Geometry check sheet. Reference: the model listing, model coordinates, mm. Face numbers are marked on the shaded views. A direction names the side the tool comes from. Coordinates: 2 decimals unless noted, no trailing zeros. Loops run counter-clockwise (first coordinate to the right, second up) from the corner with the lowest first, then second, coordinate; pieces in that order, holes last. Notation, with made-up numbers: M 63,13.25 L 119,13.25 A27 ccw 119,37.25 Z; hole C 53,-19.5 d11. An arc over 180 degrees is marked long. One line per question, with ' | ' between items. Start each with the question number.
from build123d import *

# Parameters (mm, degrees)
ESQUISSE1_R                  = 5
BOSS_EXTRU_1_DEPTH           = 10
ENL_V_MAT_EXTRU_1_DEPTH      = 3
ESQUISSE3_R                  = 2.65
ENL_V_MAT_EXTRU_2_DEPTH      = 6
ENL_V_MAT_EXTRU_3_DEPTH      = 13.247448714
ENL_V_MAT_EXTRU_3_DEPTH_BACK = 13.247448714
ESQUISSE4_R                  = 1.5
ESQUISSE5_R                  = 2.65
ENL_V_MAT_EXTRU_4_DEPTH      = 10.273618668


with BuildPart() as part:
    # Esquisse1 → Boss.-Extru.1 (new body)
    with BuildSketch(Plane.XY):
        Circle(ESQUISSE1_R)
    extrude(amount=BOSS_EXTRU_1_DEPTH)

    # Esquisse2 → Enlèv. mat.-Extru.1 (cut)
    with BuildSketch(Plane.XY.offset(10)):
        Polygon((3.7, -2.136195996), (3.7, 2.136195996), (0, 4.272391992), (-3.7, 2.136195996), (-3.7, -2.136195996), (0, -4.272391992), align=None)
    extrude(amount=-ENL_V_MAT_EXTRU_1_DEPTH, mode=Mode.SUBTRACT)

    # Esquisse3 → Enlèv. mat.-Extru.2 (cut)
    with BuildSketch(Plane(origin=(0, 0, 0), x_dir=(-1, 0, 0), z_dir=(0, 0, -1))):
        Circle(ESQUISSE3_R)
    extrude(amount=-ENL_V_MAT_EXTRU_2_DEPTH, mode=Mode.SUBTRACT)

    # Esquisse4 → Enlèv. mat.-Extru.3 (cut, two sides: drawn at the far end of the back side and taken through both)
    with BuildSketch(Plane(origin=(0, 0, 0), x_dir=(1, 0, 0), z_dir=(0, 1, 0)).offset(-ENL_V_MAT_EXTRU_3_DEPTH_BACK)):
        with Locations(Location((0, -3, 0), (0, 0, 270))):
            Circle(ESQUISSE4_R)
    extrude(amount=ENL_V_MAT_EXTRU_3_DEPTH + ENL_V_MAT_EXTRU_3_DEPTH_BACK, mode=Mode.SUBTRACT)

    # Esquisse5 → Enlèv. mat.-Extru.4 (cut, through all)
    with BuildSketch(Plane(origin=(0, 0, 6), x_dir=(-1, 0, 0), z_dir=(0, 0, -1))):
        Circle(ESQUISSE5_R)
    extrude(amount=-ENL_V_MAT_EXTRU_4_DEPTH, mode=Mode.SUBTRACT)


solid = part.part
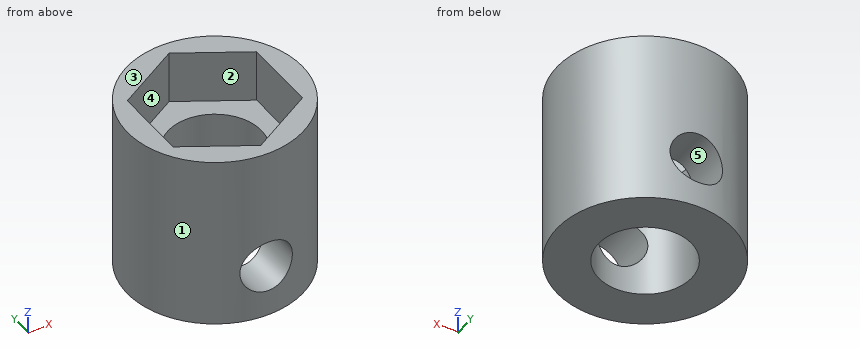
1. Tool access check on the marked faces 4 and 5. Record the directions out of +Z, -Z, +X, -X, +Y, -Y that give a thin tool (end or side, any length) a straight path to the whole face; none if there is none.
2. Sectioned sample at D-D (z = 5.5). Record the cut outline in (x, y).
3. Sectioned sample at C-C (z = 2.5). Record the cut outline in (x, y).
4. Thickness scan on line 1 (Y direction, x = 0, z = 5.75); line 2 (X direction, y = -3.25, z = 8); line 3 (X direction, y = -2, z = 6). Record the ranges inside material, lowest first.
5. Sectioned sample at A-A (y = 0). Record the cut outline in (x, z).
6. Sectioned sample at B-B (x = 2). Record the cut outline in (y, z), and give its area (3 significant figures).
7. Depth check by flat-ended pin: pin 1 Ø2 at (x, y) = (1.5, -1.5) entering from +Z; pin 2 Ø5 at (x, y) = (0, 0) entering from -Z; pin 3 Ø4 at (x, z) = (0, 3) entering from +Y; pin 4 Ø1 at (y, z) = (-2, 9) entering from -X. Enter the tip coordinate at first touch or a pass-through.
8. Draft check along Y on the marked faces 1, 2 and 3. Enter one of: +Y half, -Y half, draft (parallel to the pull), parting line (faces both ways), or undercut.
Result:
1) face 4: +Z | face 5: +Y, -Y
2) outline: C 0,0 d10; hole C 0,0 d5.3
3) outline: M -1.41,-4.8 L -1.41,-2.24 A2.65 cw -1.41,2.24 L -1.41,4.8 A5 ccw Z; M 1.41,-4.8 A5 ccw 1.41,4.8 L 1.41,2.24 A2.65 cw 1.41,-2.24 Z
4) line 1: y = -5 to -2.65, 2.65 to 5 | line 2: x = -3.8 to -1.77, 1.77 to 3.8 | line 3: x = -4.58 to -1.74, 1.74 to 4.58
5) outline: M -5,0 L -2.65,0 L -2.65,7 L -3.7,7 L -3.7,10 L -5,10 Z; M 2.65,0 L 5,0 L 5,10 L 3.7,10 L 3.7,7 L 2.65,7 Z
6) outline: M -4.58,0 L -1.74,0 L -1.74,7 L -3.12,7 L -3.12,10 L -4.58,10 Z; M 1.74,0 L 4.58,0 L 4.58,10 L 3.12,10 L 3.12,7 L 1.74,7 Z | area: 48.6 mm2
7) pin 1: stops at z = 7 | pin 2: passes through | pin 3: stops at y = 5 | pin 4: stops at x = -4.77
8) face 1: parting line | face 2: undercut | face 3: draft
